from build123d import *

# Parameters (mm, degrees)
SKETCH1_W                                = 158
SKETCH1_H                                = 25.6
PRIMARY_BACKPLATE_DEPTH                  = 1.6
SKETCH2_W                                = 172
SKETCH2_H                                = 19
PLATE_THICKENER_DEPTH                    = 1.6
SKETCH13_W                               = 9
SKETCH13_H                               = 9
THICKER_REAR_BOLT_BLOCKS_DEPTH           = 2
TAP_DRILL_FOR_M2_5X0_45_TAP3_D           = 2.05
TAP_DRILL_FOR_M2_5X0_45_TAP3_CSINK_D     = 2.1
TAP_DRILL_FOR_M2_5X0_45_TAP3_CSINK_ANGLE = 90
SKETCH7_W                                = 8
SKETCH7_H                                = 7
SKETCH7_R                                = 1.3
MOUNTING_BOSSES_DEPTH                    = 4
MOUNTING_BOSSES_2_DEPTH                  = 4
USB_HOLE_DEPTH                           = 91.001999978
USB_HOLE_DEPTH_BACK                      = 91.001999978
SKETCH8_W                                = 13.43739998
SKETCH8_H                                = 6.546680298
FILLET1_R                                = 0.5
SKETCH9_W                                = 29.257163278
SKETCH9_H                                = 15.778717932
MODULE_RELIEF_DEPTH                      = 1.6
FILLET2_R                                = 1
FILLET3_R                                = 0.75
SKETCH12_W                               = 3.613166431
SKETCH12_H                               = 1.901681258
LED_HOLE_DEPTH                           = 3


with BuildPart() as part:
    # Sketch1 → Primary backplate (new body)
    with BuildSketch(Plane.XY):
        with Locations((0, 12.8)):
            Rectangle(SKETCH1_W, SKETCH1_H)
    extrude(amount=PRIMARY_BACKPLATE_DEPTH)

    # Sketch2 → Plate thickener (add)
    with BuildSketch(Plane.XY):
        with Locations((0, 13.5)):
            Rectangle(SKETCH2_W, SKETCH2_H)
    extrude(amount=-PLATE_THICKENER_DEPTH)

    # Sketch13 → Thicker rear bolt blocks (add)
    with BuildSketch(Plane(origin=(0, 0, -1.6), x_dir=(-1, 0, 0), z_dir=(0, 0, -1))):
        with Locations((-81.5, 8.5)):
            Rectangle(SKETCH13_W, SKETCH13_H)
        with Locations((81.5, 8.5)):
            Rectangle(SKETCH13_W, SKETCH13_H)
    extrude(amount=THICKER_REAR_BOLT_BLOCKS_DEPTH)

    # Tap Drill for M2.5x0.45 Tap3 (through all)
    with Locations(Plane(origin=(-82, 9, 0), x_dir=(1, 0, 0), z_dir=(0, 0, 1))):
        with Locations((0, 0), (164, 0)):
            CounterSinkHole(TAP_DRILL_FOR_M2_5X0_45_TAP3_D / 2, TAP_DRILL_FOR_M2_5X0_45_TAP3_CSINK_D / 2, counter_sink_angle=TAP_DRILL_FOR_M2_5X0_45_TAP3_CSINK_ANGLE)

    # Sketch8 → USB hole (cut, two sides: drawn at the far end of the back side and taken through both)
    with BuildSketch(Plane.XY.offset(-USB_HOLE_DEPTH_BACK)):
        with Locations((47.742572722, 8.497650706)):
            Rectangle(SKETCH8_W, SKETCH8_H)
    extrude(amount=USB_HOLE_DEPTH + USB_HOLE_DEPTH_BACK, mode=Mode.SUBTRACT)


with BuildPart() as body_2:
    # Sketch7 → Mounting bosses (new body)
    with BuildSketch(Plane(origin=(0, 1.6, 0), x_dir=(1, 0, 0), z_dir=(0, 1, 0))):
        with Locations((-56.9, 3.5)):
            Rectangle(SKETCH7_W, SKETCH7_H)
        with Locations(Location((-56.9, 4.51, 0), (0, 0, 270))):
            Circle(SKETCH7_R, mode=Mode.SUBTRACT)
    extrude(amount=MOUNTING_BOSSES_DEPTH)


with BuildPart() as body_3:
    # Sketch7 → Mounting bosses 2 (new body)
    with BuildSketch(Plane(origin=(0, 1.6, 0), x_dir=(1, 0, 0), z_dir=(0, 1, 0))):
        with Locations((66.9, 3.5)):
            Rectangle(SKETCH7_W, SKETCH7_H)
        with Locations(Location((66.9, 4.51, 0), (0, 0, 270))):
            Circle(SKETCH7_R, mode=Mode.SUBTRACT)
    extrude(amount=MOUNTING_BOSSES_2_DEPTH)


with BuildPart() as part_1:
    add(part.part)

    # Combine1: union body 3, body 2
    add(body_3.part)
    add(body_2.part)

    # Fillet1
    fillet1_edges = [part_1.edges().sort_by_distance(p)[0] for p in [
        (-56.9, 5.6, -1.6),
        (66.9, 5.6, -1.6),
        (70.9, 4.8, -1.6),
        (62.9, 4.8, -1.6),
        (-60.9, 4.8, -1.6),
        (-52.9, 4.8, -1.6),
        (77, 8.5, -1.6),
        (81.5, 13, -1.6),
        (-81.5, 13, -1.6),
        (-77, 8.5, -1.6),
    ]]
    fillet(fillet1_edges, radius=FILLET1_R)

    # Sketch9 → module relief (cut)
    with BuildSketch(Plane(origin=(0, 0, -1.6), x_dir=(-1, 0, 0), z_dir=(0, 0, -1))):
        with Locations((-47.06304244, 8.354907592)):
            Rectangle(SKETCH9_W, SKETCH9_H)
    extrude(amount=-MODULE_RELIEF_DEPTH, mode=Mode.SUBTRACT)

    # Fillet2
    fillet2_edges = [part_1.edges().sort_by_distance(p)[0] for p in [
        (54.461272712, 11.770990855, 0.8),
        (41.023872732, 11.770990855, 0.8),
        (41.023872732, 5.224310557, 0.8),
        (54.461272712, 5.224310557, 0.8),
    ]]
    fillet(fillet2_edges, radius=FILLET2_R)

    # Fillet3
    fillet3_edges = [part_1.edges().sort_by_distance(p)[0] for p in [
        (47.742572722, 5.224310557, 1.6),
        (41.023872732, 8.497650706, 1.6),
        (54.461272712, 8.497650706, 1.6),
        (47.742572722, 11.770990855, 1.6),
        (41.31676595, 5.517203775, 1.6),
        (54.168379493, 5.517203775, 1.6),
        (54.168379493, 11.478097636, 1.6),
        (41.31676595, 11.478097636, 1.6),
    ]]
    fillet(fillet3_edges, radius=FILLET3_R)

    # Sketch12 → LED hole (cut)
    with BuildSketch(Plane(origin=(0, 0, -1.6), x_dir=(-1, 0, 0), z_dir=(0, 0, -1))):
        with Locations((-22.440360865, 2.876256908)):
            Rectangle(SKETCH12_W, SKETCH12_H)
    extrude(amount=-LED_HOLE_DEPTH, mode=Mode.SUBTRACT)


solid = part_1.part
Here's how the part is built. I have some questions about the finished solid (model axes, mm). A direction names the side the tool comes from. Give positions to 0.01 mm unless a question says otherwise; leave off trailing zeros. Order: outer loops, then holes, each group sorted by start corner. A loop starts at its lowest first (then second) coordinate and runs counter-clockwise, first axis right, second up. Notation, with made-up numbers: (-23, 47.5) -> (-18, 47.5) arc R8 ccw to (-18, 52.5) -> close; hole circle Ø5 at (87, 89). An arc over 180 degrees is marked (long way). One line per item, written item: value. Start each with the question number.
1. I need wall thicknesses on probe 1 along X at (y, z) = (4.1, -4.51); probe 2 along X at (y, z) = (9, -2.05) (1 decimal); probe 3 along X at (y, z) = (10.75, -3). Which ranges of each line are inside material? Lowest first, please. Write a range as from..to.
2. Imagine slicing it at A-A, the plane x = 26. List the corners of the cut face in (y, z) for me.
3. We'd pull the mould along X, two halves only. Please class faces 1 (the face through (86, 11, -1)), 2 (the face through (-86, 11, -1)), 3 (the face through (-76, 4, -1)), 4 (the face through (-1, 16, -1.6)): released by +X, released by -X, zero draft, split by the parting line, or undercut.
4. For faces 5 (the face through (11, 3, 0)), 6 (the face through (66, 5.6, -6)), 7 (the face through (81.6, 7.6, -3.6)), 8 (the face through (67, 1.6, -3)), which set-ups out of +Z, -Z, +X, -X, +Y, -Y let a thin tool reach every point of the face, with its end or its side?
5. Will these pins go through, and if not, where does the flat tip stop? pin 1 Ø3 at (x, z) = (66.9, -4.51) entering from +Y; pin 2 Ø1.6 at (x, z) = (-81, -3) entering from +Y; pin 3 Ø1.3 at (y, z) = (16.5, 1) entering from +X.
Values follow:
1. probe 1: x = -60.9..-58.2, -55.6..-52.9, 62.9..65.6, 68.2..70.9
1. probe 2: x = -86..-83, -81..-77, 77..81, 83..86
1. probe 3: x = -86..-77, 77..86
2. outline: (0, 0) -> (4, 0) -> (4, -1.6) -> (23, -1.6) -> (23, 0) -> (25.6, 0) -> (25.6, 1.6) -> (0, 1.6) -> close
3. face 1: released by +X
3. face 2: released by -X
3. face 3: zero draft
3. face 4: undercut
4. face 5: -Z, -Y
4. face 6: -Z, +Y
4. face 7: -Z, +X, +Y, -Y
4. face 8: -Z, +X, -X, -Y
5. pin 1: stops at y = 5.6
5. pin 2: stops at y = 13
5. pin 3: stops at x = 79
